The listing builds one solid part. Answer for the finished solid, in the listing's coordinates (mm). Face numbers are marked on the shaded views. A direction names the side the tool comes from. Give positions to 0.01 mm unless a question says otherwise; leave off trailing zeros. Order: outer loops, then holes, each group sorted by start corner. A loop starts at its lowest first (then second) coordinate and runs counter-clockwise, first axis right, second up. Notation, with made-up numbers: (26.5, 69.5) -> (37.5, 69.5) arc R29 cw to (37.5, 95.5) -> close; hole circle Ø8 at (79.25, 32). An arc over 180 degrees is marked (long way). Answer as a JSON object with one key per item and string values. Group by question number.
```python
from build123d import *

# Parameters (mm, degrees)
F1_DEPTH = 25.4
F2_T     = -2.54


with BuildPart() as f1:
    # F0 (on Front) → F1 (new body)
    with BuildSketch(Plane.XZ):
        Polygon((2.8720393181, 48.1509345859), (-44.7529606819, 48.1509345859), (-44.7529606819, 35.4509345859), (-22.5279606819, 35.4509345859), (-22.5279606819, 22.7509345859), (-9.8279606819, 10.0509345859), (2.8720393181, 22.7509345859), align=None)
        Polygon((-44.7529606819, 35.4509345859), (-44.7529606819, 48.1509345859), (-92.3779606819, 48.1509345859), (-92.3779606819, 22.7509345859), (-79.6779606819, 10.0509345859), (-66.9779606819, 22.7509345859), (-66.9779606819, 35.4509345859), align=None)
    extrude(amount=F1_DEPTH)

    # F2
    f2_openings = [f1.faces().sort_by_distance(p)[0] for p in [
        (-44.752961, -12.7, 48.150935),
    ]]
    offset(amount=F2_T, openings=f2_openings, kind=Kind.INTERSECTION)


solid = f1.part
```
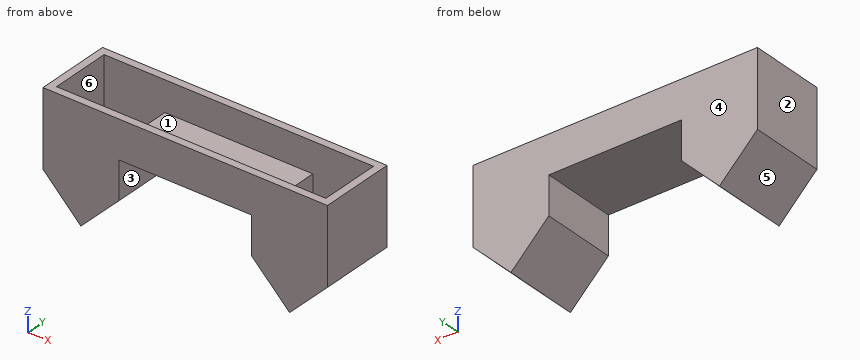
(1) A cutting plane is placed at B-B (x = -46.5). Determine the outline of the cut face in (y, z), and give its area (3 significant figures).
(2) A cutting plane is placed at D-D (y = -22). Determine the outline of the cut face in (x, z).
(3) A cutting plane is placed at C-C (z = 44.5). Determine the outline of the cut face in (x, y).
(4) Which of the six approach directions +Z, -Z, +X, -X, +Y, -Y give full straight-line access (tool end or side, diameter ignored) to the marked faces 1, 2 and 3?
(5) Flat-ended cylindrical pins translate along their axes: pin 1 Ø1.5 at (x, z) = (-25, 23) entering from +Y; pin 2 Ø7.5 at (x, y) = (-54.5, -8.5) entering from -Z; pin 3 Ø1.5 at (x, y) = (-67.5, -21.5) entering from +Z; pin 4 Ø10.5 at (x, z) = (-27, 37.5) entering from +Y. Find the tip coordinate at first contact, or state that the pin passes through.
(6) For a pull along X with two mould halves and no side action, classify the marked faces 4, 5 and 6 as +X half, -X half, draft (parallel to the pull), parting line (faces both ways), or undercut.
(7) A cutting plane is placed at A-A (z = 27). Determine the outline of the cut face in (x, y), and give its area (3 significant figures).
(8) Find the intervals of material crossed by line 1 along X through (y, z) = (-21.75, 36.5); line 2 along X through (y, z) = (-4.5, 32); line 3 along Y through (x, z) = (-10, 28), in increasing order. Write a range as [from, to].
Check sheet entries:
{
 "1": {"outline": "(-25.4, 35.45) -> (0, 35.45) -> (0, 48.15) -> (-2.54, 48.15) -> (-2.54, 37.99) -> (-22.86, 37.99) -> (-22.86, 48.15) -> (-25.4, 48.15) -> close", "area": "116 mm2"},
 "2": {"outline": "(-92.38, 22.75) -> (-79.68, 10.05) -> (-66.98, 22.75) -> (-66.98, 35.45) -> (-22.53, 35.45) -> (-22.53, 22.75) -> (-9.83, 10.05) -> (2.87, 22.75) -> (2.87, 48.15) -> (0.33, 48.15) -> (0.33, 23.8) -> (-9.83, 13.64) -> (-19.99, 23.8) -> (-19.99, 37.99) -> (-69.52, 37.99) -> (-69.52, 23.8) -> (-79.68, 13.64) -> (-89.84, 23.8) -> (-89.84, 48.15) -> (-92.38, 48.15) -> close"},
 "3": {"outline": "(-92.38, -25.4) -> (2.87, -25.4) -> (2.87, 0) -> (-92.38, 0) -> close; hole (-89.84, -22.86) -> (0.33, -22.86) -> (0.33, -2.54) -> (-89.84, -2.54) -> close"},
 "4": {"face 1": "+Z", "face 2": "+Z, -Z, -X, +Y, -Y", "face 3": "-Z, +Y, -Y"},
 "5": {"pin 1": "passes through", "pin 2": "stops at z = 35.45", "pin 3": "stops at z = 37.99", "pin 4": "stops at y = 0"},
 "6": {"face 4": "draft", "face 5": "-X half", "face 6": "undercut"},
 "7": {"outline": "(-92.38, -25.4) -> (-66.98, -25.4) -> (-66.98, 0) -> (-92.38, 0) -> close; (-22.53, -25.4) -> (2.87, -25.4) -> (2.87, 0) -> (-22.53, 0) -> close; hole (-89.84, -22.86) -> (-69.52, -22.86) -> (-69.52, -2.54) -> (-89.84, -2.54) -> close; hole (-19.99, -22.86) -> (0.33, -22.86) -> (0.33, -2.54) -> (-19.99, -2.54) -> close", "area": "465 mm2"},
 "8": {"line 1": "x = [-92.38, -89.84], [-69.52, -19.99], [0.33, 2.87]", "line 2": "x = [-92.38, -89.84], [-69.52, -66.98], [-22.53, -19.99], [0.33, 2.87]", "line 3": "y = [-25.4, -22.86], [-2.54, 0]"}
}
